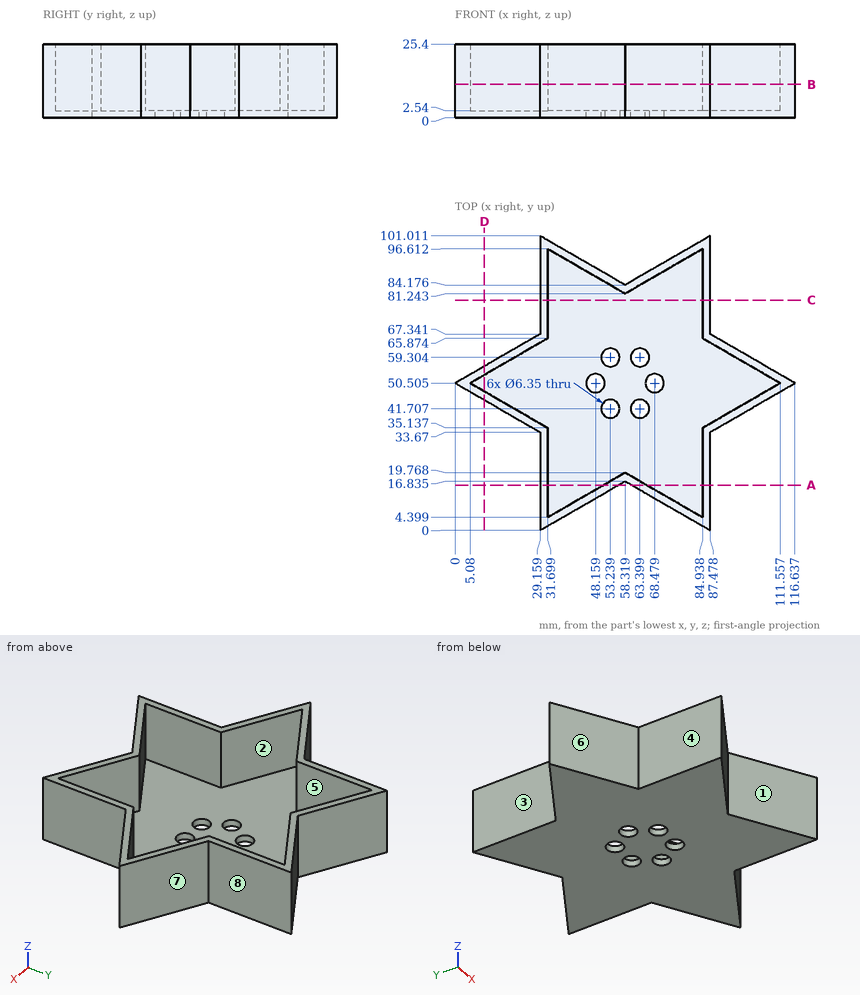
Here's the drawing with two shaded views (mm, measured from the low corner). I have some questions. A direction names the side the tool comes from. Coordinates: 2 decimals unless noted, no trailing zeros. Loops run counter-clockwise (first coordinate to the right, second up) from the corner with the lowest first, then second, coordinate; pieces in that order, holes last. Notation, with made-up numbers: M -15.5,84 L 33.5,84 A24 cw 33.5,122 Z; hole C 16.5,-18.5 d7. An arc over 180 degrees is marked long. Answer as CSV lines item,"result". Start each with the question number.
1. If I drill on probe 1 along X at (y, z) = (20.5, 23.75); probe 2 along X at (y, z) = (15, 6.75) (1 decimal); probe 3 along Y at (x, z) = (70.5, 5.5) (1 decimal), over which ranges is the centre line in solid material (lowest first)? Write a range as [from, to].
2. Suppose I cut it at A-A, the plane y = 15.5. List the corners of the cut face in (x, z) for me.
3. Suppose I cut it at B-B, the plane z = 11.5. List the corners of the cut face in (x, y) for me (1 decimal).
4. For the marked faces 1, 2, 3 and 4, which set-ups out of +Z, -Z, +X, -X, +Y, -Y let a thin tool reach every point of the face, with its end or its side?
5. Suppose I cut it at C-C, the plane y = 79. List the corners of the cut face in (x, z) for me, plus the area to 3 significant figures.
6. For pin 1 Ø4 at (x, y) = (63.4, 59.3) entering from -Z; pin 2 Ø12.5 at (y, z) = (90, 8) entering from +X; pin 3 Ø7.5 at (x, y) = (63.4, 41.71) entering from +Z; pin 4 Ø8 at (y, z) = (42, 21) entering from +X (1 decimal), each with a flat end and sliding along its axis, tell me the tip position at first contact or that it passes through.
7. Thinking about a two-plate mould opening in Y: for the marked faces 5, 6, 7 and 8, which applies, +Y half, -Y half, draft (parallel to the pull), parting line (faces both ways), or undercut?
8. Suppose I cut it at D-D, the plane x = 10. List the corners of the cut face in (y, z) for me (1 decimal).
Output:
1,probe 1,"x = [29.16, 31.7], [84.94, 87.48]"
1,probe 2,"x = [29.2, 31.7], [50.1, 55.1], [61.5, 66.6], [84.9, 87.5]"
1,probe 3,"y = [9.8, 12.7], [88.3, 91.2]"
2,outline,"M 29.16,0 L 56.01,0 L 56.01,25.4 L 50.93,25.4 L 50.93,2.54 L 31.7,2.54 L 31.7,25.4 L 29.16,25.4 Z; M 60.63,0 L 87.48,0 L 87.48,25.4 L 84.94,25.4 L 84.94,2.54 L 65.71,2.54 L 65.71,25.4 L 60.63,25.4 Z"
3,outline,"M 0,50.5 L 29.2,33.7 L 29.2,0 L 58.3,16.8 L 87.5,0 L 87.5,33.7 L 116.6,50.5 L 87.5,67.3 L 87.5,101 L 58.3,84.2 L 29.2,101 L 29.2,67.3 Z; hole M 5.1,50.5 L 31.7,35.1 L 31.7,4.4 L 58.3,19.8 L 84.9,4.4 L 84.9,35.1 L 111.6,50.5 L 84.9,65.9 L 84.9,96.6 L 58.3,81.2 L 31.7,96.6 L 31.7,65.9 Z"
4,face 1,"+Z, -Z, -Y"
4,face 2,"+Z"
4,face 3,"+Z, -Z, -X, +Y"
4,face 4,"+Z, -Z, -X, -Y"
5,outline,"M 29.16,0 L 87.48,0 L 87.48,25.4 L 84.94,25.4 L 84.94,2.54 L 31.7,2.54 L 31.7,25.4 L 29.16,25.4 Z"
5,area,"264 mm^2"
6,pin 1,"passes through"
6,pin 2,"stops at x = 87.48"
6,pin 3,"stops at z = 2.54"
6,pin 4,"stops at x = 108.8"
7,face 5,"undercut"
7,face 6,"-Y half"
7,face 7,"+Y half"
7,face 8,"draft"
8,outline,"M 44.7,0 L 56.3,0 L 56.3,25.4 L 53.3,25.4 L 53.3,2.5 L 47.7,2.5 L 47.7,25.4 L 44.7,25.4 Z"
